from build123d import *

# Parameters (mm, degrees)
SKETCH1_W               = 50
SKETCH1_H               = 156
BOSS_EXTRUDE1_DEPTH     = 5
CUT_EXTRUDE1_DEPTH      = 22.86
CUT_EXTRUDE1_DEPTH_BACK = 20.32
SKETCH2_W               = 25
SKETCH2_H               = 3


with BuildPart() as part:
    # Sketch1 → Boss-Extrude1 (new body)
    with BuildSketch(Plane.XY):
        Rectangle(SKETCH1_W, SKETCH1_H)
    extrude(amount=BOSS_EXTRUDE1_DEPTH)

    # Sketch2 → Cut-Extrude1 (cut, two sides: drawn at the far end of the back side and taken through both)
    with BuildSketch(Plane.XY.offset(5).offset(-CUT_EXTRUDE1_DEPTH_BACK)):
        with Locations((0, 76.5)):
            Rectangle(SKETCH2_W, SKETCH2_H)
        with Locations((0, -76.5)):
            Rectangle(SKETCH2_W, SKETCH2_H)
    extrude(amount=CUT_EXTRUDE1_DEPTH + CUT_EXTRUDE1_DEPTH_BACK, mode=Mode.SUBTRACT)


solid = part.part
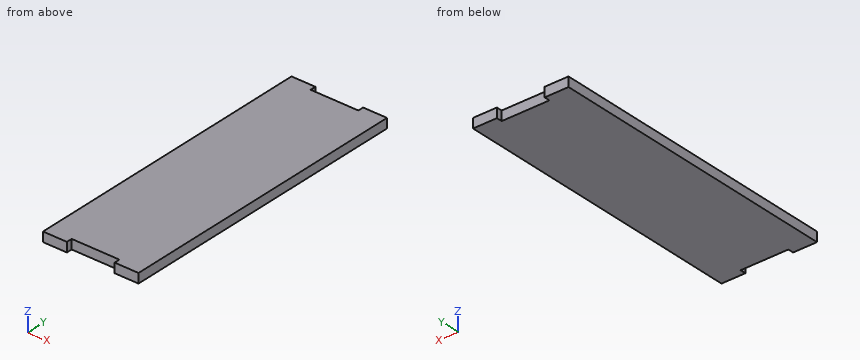
Input: part model. Units: mm. Frame: model coordinates. Round coordinates to 2 decimals unless told otherwise and drop trailing zeros. Order: outer loops, then holes, each group sorted by start corner. A loop starts at its lowest first (then second) coordinate and runs counter-clockwise, first axis right, second up. Notation, with made-up numbers: (82.25, -11) - (118.25, -11) arc R18 ccw to (118.25, -3) - close; hole circle Ø7 at (-16, 79.5). An arc over 180 degrees is marked (long way). Answer as a JSON object with one key per item and string values. Group by question number.
(1) Pin query (flat end, axial travel): P1, Ø2.5, axis at x = -2.5, z = 3, coming from the -Y side; P2, Ø2.5, axis at x = 1, z = 2, coming from the +Y side. Return the tip coordinate at first contact, or that it passes through.
(2) Material intervals for probe 1 along Y at (x, z) = (6.5, 2.45), sorted ascending. Write a range as from..to.
(3) Cut plane A-A (z = 0.75). Return loops of the section in (x, y).
(4) Cut plane B-B (x = -10.5). Return loops of the section in (y, z).
Here are the results:
{
 "1": {"P1": "stops at y = -75", "P2": "stops at y = 75"},
 "2": {"probe 1": "y = -75..75"},
 "3": {"outline": "(-25, -78) - (-12.5, -78) - (-12.5, -75) - (12.5, -75) - (12.5, -78) - (25, -78) - (25, 78) - (12.5, 78) - (12.5, 75) - (-12.5, 75) - (-12.5, 78) - (-25, 78) - close"},
 "4": {"outline": "(-75, 0) - (75, 0) - (75, 5) - (-75, 5) - close"}
}
